```python
from build123d import *

# Parameters (mm, degrees)
F1_DEPTH = 6.35


with BuildPart() as f1:
    # F0 (on Front) → F1 (new body)
    with BuildSketch(Plane.XZ):
        Polygon((0, 10), (0, 0), (15, 0), (15, 6.35), (18.5, 6.35), (18.5, 14), (17.3, 14), (17.3, 16.27), (18.5, 16.27), (18.5, 20), (21.5, 20), (21.5, 16.27), (22.7, 16.27), (22.7, 14), (21.5, 14), (21.5, 6.35), (25, 6.35), (25, 0), (102.3, 0), (102.3, 6.35), (105.8, 6.35), (105.8, 14), (104.6, 14), (104.6, 16.27), (105.8, 16.27), (105.8, 20), (108.8, 20), (108.8, 16.27), (110, 16.27), (110, 14), (108.8, 14), (108.8, 6.35), (112.3, 6.35), (112.3, 0), (127.3, 0), (127.3, 10), (133.65, 10), (133.65, 20), (127.3, 20), (127.3, 35), (133.65, 35), (133.65, 45), (127.3, 45), (127.3, 55), (106.15, 55), (106.15, 61.35), (96.15, 61.35), (96.15, 55), (81.15, 55), (81.15, 61.35), (71.15, 61.35), (71.15, 55), (56.15, 55), (56.15, 61.35), (46.15, 61.35), (46.15, 55), (31.15, 55), (31.15, 61.35), (21.15, 61.35), (21.15, 55), (0, 55), (0, 45), (-6.35, 45), (-6.35, 35), (0, 35), (0, 20), (-6.35, 20), (-6.35, 10), align=None)
        with BuildLine():
            ThreePointArc((35, 12.3), (36.464466, 15.835534), (40, 17.3))
            Line((40, 17.3), (87.3, 17.3))
            ThreePointArc((87.3, 17.3), (90.835534, 15.835534), (92.3, 12.3))
            Line((92.3, 12.3), (92.3, 11.35))
            ThreePointArc((92.3, 11.35), (90.835534, 7.814466), (87.3, 6.35))
            Line((87.3, 6.35), (40, 6.35))
            ThreePointArc((40, 6.35), (36.464466, 7.814466), (35, 11.35))
            Line((35, 11.35), (35, 12.3))
        make_face(mode=Mode.SUBTRACT)
        with BuildLine():
            ThreePointArc((15, 43.65), (16.464466, 47.185534), (20, 48.65))
            Line((20, 48.65), (107.3, 48.65))
            ThreePointArc((107.3, 48.65), (110.835534, 47.185534), (112.3, 43.65))
            Line((112.3, 43.65), (112.3, 28.65))
            ThreePointArc((112.3, 28.65), (110.835534, 25.114466), (107.3, 23.65))
            Line((107.3, 23.65), (20, 23.65))
            ThreePointArc((20, 23.65), (16.464466, 25.114466), (15, 28.65))
            Line((15, 28.65), (15, 43.65))
        make_face(mode=Mode.SUBTRACT)
    extrude(amount=F1_DEPTH)


solid = f1.part
```
Verification items for the finished model (mm, model axes). A direction names the side the tool comes from. Coordinates: 2 decimals unless noted, no trailing zeros. Loops run counter-clockwise (first coordinate to the right, second up) from the corner with the lowest first, then second, coordinate; pieces in that order, holes last. Notation, with made-up numbers: (75, -11.75) -> (118, -11.75) arc R31 cw to (118, 14.25) -> close; hole circle Ø10 at (11, 71). An arc over 180 degrees is marked (long way). Answer in a Markdown table with one row per item. Add a question column.
1. Section check D-D, the plane y = -5. Give the number of separate pieces and of enclosed holes in the cut face, then the cut area to 3 significant figures.
2. Material ranges on probe 1 along Z at (x, y) = (49.5, -2.5); probe 2 along Z at (x, y) = (71, -4.5); probe 3 along X at (y, z) = (-3.75, 56.5), recorded low to high. Write a range as [from, to].
3. Section check A-A, the plane x = 100. Enter the section's corners in (y, z), then the cut area to 3 significant figures.
4. Section check B-B, the plane z = 33.5. Enter the section's corners in (x, y).
5. Section check C-C, the plane x = 59. Enter the section's corners in (y, z).
6. Draft check along Z on faces 1 (the face through (16.43, -3.13, 47.15)), 2 (the face through (-6.35, -3, 15)), 3 (the face through (20, -3, 20)). Enter one of: +Z half, -Z half, draft (parallel to the pull), parting line (faces both ways), or undercut.
7. Access from +Z, -Z, +X, -X, +Y, -Y to the whole of each face (thin tool, end or side, straight path). Record for faces 4 (the face through (90.87, -3.13, 7.85)), 5 (the face through (46.15, -3, 58)), 6 (the face through (18.5, -3, 18)).
8. Depth check by flat-ended pin: P1, Ø1.9, axis at y = -2.5, z = 6.5, coming from the +X side; P2, Ø1.9, axis at x = 132, y = -4.5, coming from the -Z side; P3, Ø1.5, axis at x = 17, z = 40, coming from the -Y side; P4, Ø0.6, axis at x = 105.5, y = -3.5, coming from the -Z side. Enter the tip coordinate at first touch or a pass-through.
Derived:
| question | item | result |
|---|---|---|
| 1 | separate pieces | 1 |
| 1 | enclosed holes | 2 |
| 1 | area | 4,270 mm² |
| 2 | probe 1 | z = [0, 6.35], [17.3, 23.65], [48.65, 61.35] |
| 2 | probe 2 | z = [0, 6.35], [17.3, 23.65], [48.65, 55] |
| 2 | probe 3 | x = [21.15, 31.15], [46.15, 56.15], [71.15, 81.15], [96.15, 106.15] |
| 3 | outline | (-6.35, 0) -> (0, 0) -> (0, 23.65) -> (-6.35, 23.65) -> close; (-6.35, 48.65) -> (0, 48.65) -> (0, 61.35) -> (-6.35, 61.35) -> close |
| 3 | area | 231 mm² |
| 4 | outline | (0, -6.35) -> (15, -6.35) -> (15, 0) -> (0, 0) -> close; (112.3, -6.35) -> (127.3, -6.35) -> (127.3, 0) -> (112.3, 0) -> close |
| 5 | outline | (-6.35, 0) -> (0, 0) -> (0, 6.35) -> (-6.35, 6.35) -> close; (-6.35, 17.3) -> (0, 17.3) -> (0, 23.65) -> (-6.35, 23.65) -> close; (-6.35, 48.65) -> (0, 48.65) -> (0, 55) -> (-6.35, 55) -> close |
| 6 | face 1 | undercut |
| 6 | face 2 | draft |
| 6 | face 3 | -Z half |
| 7 | face 4 | +Y, -Y |
| 7 | face 5 | +Z, +Y, -Y |
| 7 | face 6 | -Z, +Y, -Y |
| 8 | P1 | stops at x = 127.3 |
| 8 | P2 | stops at z = 10 |
| 8 | P3 | passes through |
| 8 | P4 | stops at z = 6.35 |
